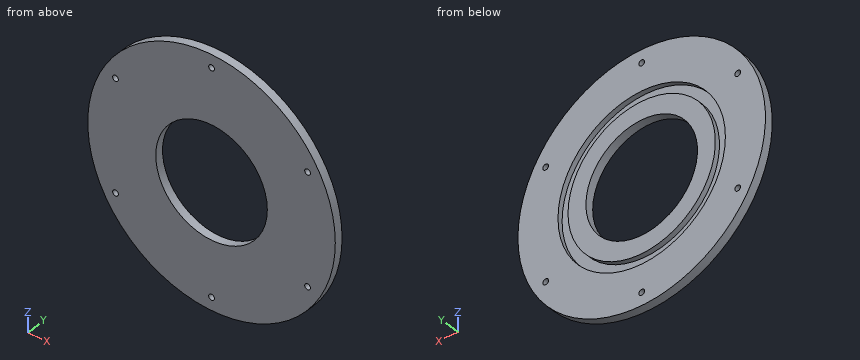
```python
from build123d import *

# Parameters (mm, degrees)
SKETCH1_R           = 86.5
SKETCH1_R_2         = 39
BOSS_EXTRUDE1_DEPTH = 5.8
SKETCH2_R           = 58.5
SKETCH2_R_2         = 51.5
CUT_EXTRUDE1_DEPTH  = 3.5
SKETCH3_R           = 2
CUT_EXTRUDE2_DEPTH  = 6.8


with BuildPart() as part:
    # Sketch1 → Boss-Extrude1 (new body)
    with BuildSketch(Plane(origin=(0, 0, 0), x_dir=(1, 0, 0), z_dir=(0, 1, 0))):
        Circle(SKETCH1_R)
        Circle(SKETCH1_R_2, mode=Mode.SUBTRACT)
    extrude(amount=BOSS_EXTRUDE1_DEPTH)

    # Sketch2 → Cut-Extrude1 (cut)
    with BuildSketch(Plane(origin=(0, 5.8, 0), x_dir=(1, 0, 0), z_dir=(0, 1, 0))):
        Circle(SKETCH2_R)
        Circle(SKETCH2_R_2, mode=Mode.SUBTRACT)
    extrude(amount=-CUT_EXTRUDE1_DEPTH, mode=Mode.SUBTRACT)

    # Sketch3 → Cut-Extrude2 (cut, through all)
    with BuildSketch(Plane(origin=(0, 5.8, 0), x_dir=(1, 0, 0), z_dir=(0, 1, 0))):
        with Locations((0, 77.5)):
            Circle(SKETCH3_R)
        with Locations((67.116968793, 38.75)):
            Circle(SKETCH3_R)
        with Locations((67.116968793, -38.75)):
            Circle(SKETCH3_R)
        with Locations((0, -77.5)):
            Circle(SKETCH3_R)
        with Locations((-67.116968793, -38.75)):
            Circle(SKETCH3_R)
        with Locations((-67.116968793, 38.75)):
            Circle(SKETCH3_R)
    extrude(amount=-CUT_EXTRUDE2_DEPTH, mode=Mode.SUBTRACT)


solid = part.part
```
CAD build for the part. Positions are in the model's coordinates, mm. Give positions to 0.01 mm unless a question says otherwise; leave off trailing zeros. Order: outer loops, then holes, each group sorted by start corner. A loop starts at its lowest first (then second) coordinate and runs counter-clockwise, first axis right, second up.
(1) Drill centre lines: L1, parallel to Z at x = 0, y = 2.1; L2, parallel to Z at x = -30.5, y = 4.2; L3, parallel to Z at x = 68, y = 4.95. Where is each one in solid material? Low to high.
(2) Flat gauge pins, fed straight in: pin 1 (3 mm diameter, centred on x = 67.12, z = 38.75, fed in from +Y); pin 2 (3 mm diameter, centred on y = 5, z = -4, fed in from -X); pin 3 (1.5 mm diameter, centred on y = 4, z = 21, fed in from +X). Where does each tip first touch, or does it go through?
(3) Saw through at C-C, the plane z = 0. Give the cut face in (x, y).
(4) Saw through at B-B, the plane x = 0. Give the cut face in (y, z).
(5) Saw through at A-A, the plane y = 3.5. State how many separate pieces and enclosed holes the cut face has, then the cut area to 3 significant figures.
(6) Saw through at D-D, the plane x = 27. Give the cut face in (y, z), then the cut area to 3 significant figures.
Results found:
1. L1: z = -86.5 to -79.5, -75.5 to -39, 39 to 75.5, 79.5 to 86.5
1. L2: z = -80.94 to -49.92, -41.5 to -24.31, 24.31 to 41.5, 49.92 to 80.94
1. L3: z = -53.46 to -40.54, -36.96 to 36.96, 40.54 to 53.46
2. pin 1: passes through
2. pin 2: stops at x = -86.46
2. pin 3: stops at x = 84.1
3. outline: (-86.5, 0) - (-39, 0) - (-39, 5.8) - (-51.5, 5.8) - (-51.5, 2.3) - (-58.5, 2.3) - (-58.5, 5.8) - (-86.5, 5.8) - close; (39, 0) - (86.5, 0) - (86.5, 5.8) - (58.5, 5.8) - (58.5, 2.3) - (51.5, 2.3) - (51.5, 5.8) - (39, 5.8) - close
4. outline: (0, -86.5) - (5.8, -86.5) - (5.8, -79.5) - (0, -79.5) - close; (0, -75.5) - (5.8, -75.5) - (5.8, -58.5) - (2.3, -58.5) - (2.3, -51.5) - (5.8, -51.5) - (5.8, -39) - (0, -39) - close; (0, 39) - (5.8, 39) - (5.8, 51.5) - (2.3, 51.5) - (2.3, 58.5) - (5.8, 58.5) - (5.8, 75.5) - (0, 75.5) - close; (0, 79.5) - (5.8, 79.5) - (5.8, 86.5) - (0, 86.5) - close
5. separate pieces: 2
5. enclosed holes: 8
5. area: 16,200 mm2
6. outline: (0, -82.18) - (5.8, -82.18) - (5.8, -51.9) - (2.3, -51.9) - (2.3, -43.85) - (5.8, -43.85) - (5.8, -28.14) - (0, -28.14) - close; (0, 28.14) - (5.8, 28.14) - (5.8, 43.85) - (2.3, 43.85) - (2.3, 51.9) - (5.8, 51.9) - (5.8, 82.18) - (0, 82.18) - close
6. area: 571 mm2
